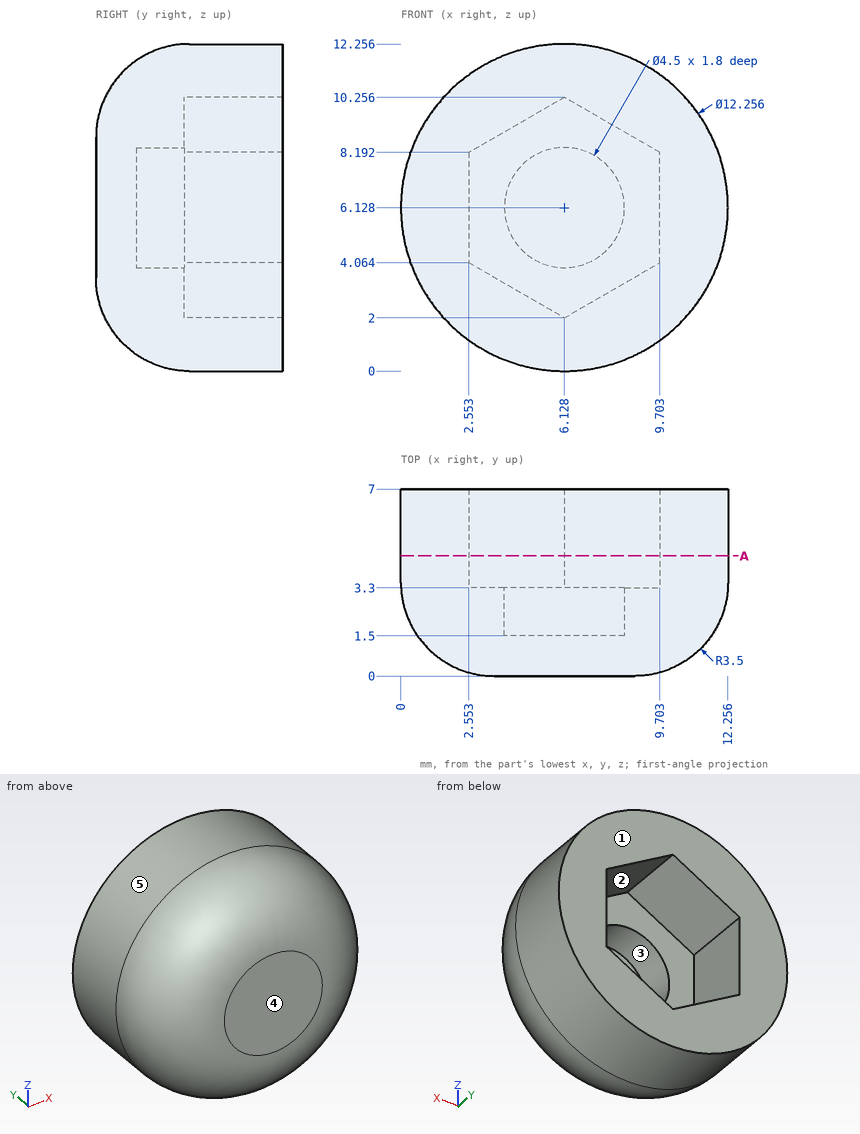
Geometry check sheet. Reference: drawing and pictorial views, mm from the part's lowest x, y, z. A direction names the side the tool comes from. Coordinates: 2 decimals unless noted, no trailing zeros. Order: outer loops, then holes, each group sorted by start corner. A loop starts at its lowest first (then second) coordinate and runs counter-clockwise, first axis right, second up.
Item 1: Release check for a two-part mould opening along Z. For the marked faces 3, 4 and 5 record: +Z half, -Z half, draft (parallel to the pull), parting line (faces both ways), or undercut.
Filled in:
face 3: undercut
face 4: draft
face 5: parting line
Item 2: Material ranges on L1, parallel to X at y = 3.75, z = 6.25 (3 decimals); L2, parallel to Z at x = 5.5, y = 5.5; L3, parallel to Z at x = 3.5, y = 4.75, recorded low to high.
Filled in:
L1: x = 0.001 to 2.553, 9.703 to 12.255
L2: z = 0.03 to 2.36, 9.89 to 12.22
L3: z = 0.59 to 3.52, 8.74 to 11.66
Item 3: Access from +Z, -Z, +X, -X, +Y, -Y to the whole of each face (thin tool, end or side, straight path). Record for the marked faces 1 and 2.
Filled in:
face 1: +Z, -Z, +X, -X, +Y
face 2: +Y
Item 4: Section check A-A, the plane y = 4.5. Enter the section's corners in (x, z).
Filled in:
outline: circle Ø12.26 at (6.13, 6.13); hole (2.55, 4.06) - (6.13, 2) - (9.7, 4.06) - (9.7, 8.19) - (6.13, 10.26) - (2.55, 8.19) - close
Item 5: Depth check by flat-ended pin: pin 1 (3.5 mm diameter, centred on x = 6.5, z = 7.5, fed in from +Y); pin 2 (1.5 mm diameter, centred on x = 1.5, y = 1.5, fed in from +Z); pin 3 (2 mm diameter, centred on x = 10, y = 1, fed in from +Z). Enter the tip coordinate at first touch or a pass-through.
Filled in:
pin 1: stops at y = 3.3
pin 2: stops at z = 10.25
pin 3: stops at z = 10.79
